```python
from build123d import *

# Parameters (mm, degrees)
SKETCH1_R                = 33.6
SKETCH1_W                = 12.6
SKETCH1_H                = 20.6
BOSS_EXTRUDE1_DEPTH      = 96
CUT_EXTRUDE1_DEPTH       = 115.550093395
CUT_EXTRUDE1_DEPTH_BACK  = 115.550093395
SKETCH2_W                = 48
SKETCH2_H                = 0.5
BOSS_EXTRUDE2_REACH      = 130.771
BOSS_EXTRUDE2_END_RADIUS = 33.6
SKETCH3_R                = 3
SKETCH4_R                = 3
CUT_EXTRUDE2_DEPTH       = 10.2
SKETCH5_R                = 1.8
CUT_EXTRUDE3_DEPTH       = 136.732562696
CIRPATTERN1_COUNT        = 4
SKETCH12_R               = 1.8
CUT_EXTRUDE7_DEPTH       = 120.152901457
CUT_EXTRUDE8_DEPTH       = 115.55009351
CUT_EXTRUDE8_DEPTH_BACK  = 115.55009351
SKETCH13_W               = 12
SKETCH13_H               = 29.4
CUT_EXTRUDE10_DEPTH      = 29.7


with BuildPart() as part:
    # Sketch1 → Boss-Extrude1 (new body)
    with BuildSketch(Plane.XY):
        with BuildLine():
            Line((-51.085456803, 12.7), (-33.685456803, 12.7))
            ThreePointArc((-33.685456803, 12.7), (36, 0), (-33.685456803, -12.7))
            Line((-33.685456803, -12.7), (-51.085456803, -12.7))
            Line((-51.085456803, -12.7), (-51.085456803, 12.7))
        make_face()
        Circle(SKETCH1_R, mode=Mode.SUBTRACT)
        with Locations((-42.385456803, 0)):
            Rectangle(SKETCH1_W, SKETCH1_H, mode=Mode.SUBTRACT)
    extrude(amount=BOSS_EXTRUDE1_DEPTH)

    # Sketch2 → Cut-Extrude1 (cut, two sides: drawn at the far end of the back side and taken through both)
    with BuildSketch(Plane(origin=(0, 0, 0), x_dir=(0, 0, -1), z_dir=(0, 1, 0)).offset(-CUT_EXTRUDE1_DEPTH_BACK)):
        with Locations((-24, 0)):
            Rectangle(SKETCH2_W, SKETCH2_H)
    extrude(amount=CUT_EXTRUDE1_DEPTH + CUT_EXTRUDE1_DEPTH_BACK, mode=Mode.SUBTRACT)

    # Boss-Extrude2: up to this cylinder (the profile starts inside it)
    boss_extrude2_end = Plane(origin=(0, 0, 12), z_dir=(0, 0, -1)) * Cylinder(BOSS_EXTRUDE2_END_RADIUS, 329.742, mode=Mode.PRIVATE)
    # Sketch3 → Boss-Extrude2 (add, up to the surface)
    with BuildSketch(Plane(origin=(16.674534964, 16.674534964, 0), x_dir=(0, 0, -1), z_dir=(0.7071067811865488, 0.7071067811865464, 0)), mode=Mode.PRIVATE) as boss_extrude2_sk1:
        with Locations(Location((-12, 0, 0), (0, 0, 270))):
            Circle(SKETCH3_R)
    boss_extrude2_tool1 = extrude(boss_extrude2_sk1.sketch, amount=BOSS_EXTRUDE2_REACH, mode=Mode.PRIVATE) & boss_extrude2_end
    add(boss_extrude2_tool1.solids().sort_by_distance((16.674535, 16.674535, 12))[0])

    # Sketch4 → Cut-Extrude2 (cut)
    with BuildSketch(Plane(origin=(16.674534964, 16.674534964, 0), x_dir=(0, 0, 1), z_dir=(-0.7071067811865487, -0.7071067811865465, 0))):
        with Locations(Location((12, 0, 0), (0, 0, 270))):
            Circle(SKETCH4_R)
    cut_extrude2 = extrude(amount=-CUT_EXTRUDE2_DEPTH, mode=Mode.SUBTRACT)

    # Sketch5 → Cut-Extrude3 (cut, through all)
    with BuildSketch(Plane(origin=(23.887024132, 23.887024132, 0), x_dir=(0, 0, 1), z_dir=(-0.7071067811865486, -0.7071067811865465, 0))):
        with Locations(Location((12, 0, 0), (0, 0, 270))):
            Circle(SKETCH5_R)
    cut_extrude3 = extrude(amount=-CUT_EXTRUDE3_DEPTH, mode=Mode.SUBTRACT)

    # CirPattern1: Cut-Extrude2, Cut-Extrude3 ×4 about axis
    cirpattern1_axis = Axis((0, 0, 0), (0, 0, 1))
    add([cut_extrude2.rotate(cirpattern1_axis, i * 360 / CIRPATTERN1_COUNT) for i in range(1, CIRPATTERN1_COUNT)], mode=Mode.SUBTRACT)
    add([cut_extrude3.rotate(cirpattern1_axis, i * 360 / CIRPATTERN1_COUNT) for i in range(1, CIRPATTERN1_COUNT)], mode=Mode.SUBTRACT)

    # Sketch12 → Cut-Extrude7 (cut, through all)
    with BuildSketch(Plane(origin=(0, 12.7, 0), x_dir=(1, 0, 0), z_dir=(0, 1, 0))):
        with Locations(Location((-42.385456803, -24, 0), (0, 0, 270))):
            Circle(SKETCH12_R)
        with Locations(Location((-42.385456803, -72, 0), (0, 0, 270))):
            Circle(SKETCH12_R)
    extrude(amount=-CUT_EXTRUDE7_DEPTH, mode=Mode.SUBTRACT)

    # Sketch13 → Cut-Extrude8 (cut, two sides: drawn at the far end of the back side and taken through both)
    with BuildSketch(Plane(origin=(0, 0, 0), x_dir=(1, 0, 0), z_dir=(0, 1, 0)).offset(-CUT_EXTRUDE8_DEPTH_BACK)):
        with Locations((0, -14.7)):
            Rectangle(SKETCH13_W, SKETCH13_H)
    extrude(amount=CUT_EXTRUDE8_DEPTH + CUT_EXTRUDE8_DEPTH_BACK, mode=Mode.SUBTRACT)

    # Sketch15 → Cut-Extrude10 (cut)
    with BuildSketch(Plane(origin=(0, 0, 0), x_dir=(-1, 0, 0), z_dir=(0, 0, -1))):
        with BuildLine():
            Line((-7.023251593, -35.308270095), (-6.55503482, -32.954385422))
            ThreePointArc((-6.55503482, -32.954385422), (0, -33.6), (6.55503482, -32.954385422))
            Line((6.55503482, -32.954385422), (7.023251593, -35.308270095))
            ThreePointArc((7.023251593, -35.308270095), (0, -36), (-7.023251593, -35.308270095))
        make_face()
        with BuildLine():
            Line((7.023251593, 35.308270095), (6.55503482, 32.954385422))
            ThreePointArc((6.55503482, 32.954385422), (0, 33.6), (-6.55503482, 32.954385422))
            Line((-6.55503482, 32.954385422), (-7.023251593, 35.308270095))
            ThreePointArc((-7.023251593, 35.308270095), (0, 36), (7.023251593, 35.308270095))
        make_face()
    extrude(amount=-CUT_EXTRUDE10_DEPTH, mode=Mode.SUBTRACT)


solid = part.part
```
CAD build for the part. Positions are in the model's coordinates, mm. A direction names the side the tool comes from. Coordinates: 2 decimals unless noted, no trailing zeros. Order: outer loops, then holes, each group sorted by start corner. A loop starts at its lowest first (then second) coordinate and runs counter-clockwise, first axis right, second up. Notation, with made-up numbers: (2.25, 76) - (51.25, 76) arc R9 ccw to (51.25, 91) - close; hole circle Ø1 at (56, 41.5). An arc over 180 degrees is marked (long way). Use a Markdown table: item, result. Add a question column.
(1) Flat gauge pins, fed straight in: pin 1 (2.5 mm diameter, centred on y = 34.5, z = 38, fed in from -X); pin 2 (2 mm diameter, centred on x = -28, z = 42, fed in from +Y); pin 3 (2 mm diameter, centred on x = 7.5, z = 49.5, fed in from +Y). Where does each tip first touch, or does it go through?
(2) Saw through at A-A (y = 0). Give the cut face in (x, z), then the cut area to 3 significant figures.
(3) Drill centre lines: line 1 along X through (y, z) = (0, 23); line 2 along X through (y, z) = (5, 49.5); line 3 along Y through (x, z) = (-48, 10.5). Where is each one in solid material? Low to high. Write a range as [from, to].
(4) Saw through at D-D (x = -1.5). Give the cut face in (y, z).
(5) Saw through at B-B (z = 72). Give the cut face in (x, y).
(6) Saw through at C-C (z = 24). Give the cut face in (x, y), then the cut area to 3 significant figures.
(7) Pull direction Y, two halves, no side cores. Call faces 1 (the face through (35.973, 1.401, 47.328)), 2 (the face through (6.786, 34.115, 14.642)), 3 (the face through (-25.272, -22.503, 12.042)), 4 (the face through (-48.685, 0, 47)): +Y half, -Y half, draft (parallel to the pull), parting line (faces both ways), or undercut.
(8) Which spindle directions (+Z, -Z, +X, -X, +Y, -Y) get a long thin tool onto all of the face, cutting with end or side? Do faces 5 (the face through (-6.792, 34.148, 14.642)), 6 (the face through (-42, -12.7, 47)), 7 (the face through (-0.25, -35, 39)), 8 (the face through (23.857, 23.917, 10.042)). Say none if no direction does.
Solved:
| question | item | result |
|---|---|---|
| 1 | pin 1 | stops at x = -13.8 |
| 1 | pin 2 | stops at y = 23.81 |
| 1 | pin 3 | stops at y = 35.41 |
| 2 | outline | (-51.09, 0) - (-48.69, 0) - (-48.69, 96) - (-51.09, 96) - close; (-36.09, 0) - (-33.6, 0) - (-33.6, 96) - (-36.09, 96) - close; (33.6, 0) - (36, 0) - (36, 96) - (33.6, 96) - close |
| 2 | area | 699 mm² |
| 3 | line 1 | x = [-51.09, -48.69], [-36.09, -33.6], [33.6, 36] |
| 3 | line 2 | x = [-51.09, -48.69], [-36.09, -33.23], [33.23, 35.65] |
| 3 | line 3 | y = [-12.7, -10.3], [10.3, 12.7] |
| 4 | outline | (-35.97, 29.7) - (-33.57, 29.7) - (-33.57, 96) - (-35.97, 96) - close; (33.57, 29.7) - (35.97, 29.7) - (35.97, 96) - (33.57, 96) - close |
| 5 | outline | (-51.09, -12.7) - (-44.19, -12.7) - (-44.19, -10.3) - (-48.69, -10.3) - (-48.69, 10.3) - (-44.19, 10.3) - (-44.19, 12.7) - (-51.09, 12.7) - close; (-40.59, -12.7) - (-33.69, -12.7) arc R36 ccw (long way) to (-33.69, 12.7) - (-40.59, 12.7) - (-40.59, 10.3) - (-36.09, 10.3) - (-36.09, -10.3) - (-40.59, -10.3) - close; hole circle Ø67.2 at (0, 0) |
| 6 | outline | (-51.09, -12.7) - (-44.19, -12.7) - (-44.19, -10.3) - (-48.69, -10.3) - (-48.69, 10.3) - (-44.19, 10.3) - (-44.19, 12.7) - (-51.09, 12.7) - close; (-40.59, -12.7) - (-33.69, -12.7) arc R36 ccw to (-7.02, -35.31) - (-6.56, -32.95) arc R33.6 cw to (-6.56, 32.95) - (-7.02, 35.31) arc R36 ccw to (-33.69, 12.7) - (-40.59, 12.7) - (-40.59, 10.3) - (-36.09, 10.3) - (-36.09, -10.3) - (-40.59, -10.3) - close; (6.56, -32.95) - (7.02, -35.31) arc R36 ccw to (7.02, 35.31) - (6.56, 32.95) arc R33.6 cw to start |
| 6 | area | 585 mm² |
| 7 | face 1 | parting line |
| 7 | face 2 | +Y half |
| 7 | face 3 | undercut |
| 7 | face 4 | undercut |
| 8 | face 5 | -Z, +Y |
| 8 | face 6 | +Z, -Z, -X, -Y |
| 8 | face 7 | -Z, +Y, -Y |
| 8 | face 8 | none |
